```python
from build123d import *

# Parameters (mm, degrees)
SKETCH_1_W          = 65
SKETCH_1_H          = 70
EXTRUDE_1_DEPTH     = 4
SKETCH_2_R          = 2.1
SKETCH_2_R_2        = 1.575
SKETCH_2_R_3        = 14
CUT_EXTRUDE_1_DEPTH = 96.608577021
CUT_EXTRUDE_2_DEPTH = 96.608577021
FILLET_1_R          = 10


with BuildPart() as part:
    # 草图1 → 凸台-拉伸1 (new body)
    with BuildSketch(Plane.XY):
        with Locations((32.5, -35)):
            Rectangle(SKETCH_1_W, SKETCH_1_H)
    extrude(amount=EXTRUDE_1_DEPTH)

    # 草图2 → 切除-拉伸1 (cut, through all)
    with BuildSketch(Plane.XY.offset(4)):
        with Locations((25, -29.5)):
            Circle(SKETCH_2_R)
        with Locations((7.5, -47)):
            Circle(SKETCH_2_R)
        with Locations(Location((25, -64.5, 0), (0, 0, 180))):
            Circle(SKETCH_2_R)
        with Locations(Location((42.5, -47, 0), (0, 0, 180))):
            Circle(SKETCH_2_R)
        with Locations((40, -5)):
            Circle(SKETCH_2_R_2)
        with Locations(Location((50, -5, 0), (0, 0, 180))):
            Circle(SKETCH_2_R_2)
        with Locations((50, -15)):
            Circle(SKETCH_2_R_2)
        with Locations(Location((40, -15, 0), (0, 0, 180))):
            Circle(SKETCH_2_R_2)
        with Locations((25, -47)):
            Circle(SKETCH_2_R_3)
    extrude(amount=-CUT_EXTRUDE_1_DEPTH, mode=Mode.SUBTRACT)

    # 草图3 → 切除-拉伸2 (cut, through all)
    with BuildSketch(Plane(origin=(0, 0, 0), x_dir=(-1, 0, 0), z_dir=(0, 0, -1))):
        Polygon((-15, 0), (0, 0), (0, -35), align=None)
        Polygon((-65, 0), (-58, 0), (-65, -40), align=None)
    extrude(amount=-CUT_EXTRUDE_2_DEPTH, mode=Mode.SUBTRACT)

    # 圆角1
    fillet_1_edges = [part.edges().sort_by_distance(p)[0] for p in [
        (0, -35, 2),
        (15, 0, 2),
        (65, -40, 2),
        (58, 0, 2),
    ]]
    fillet(fillet_1_edges, radius=FILLET_1_R)


solid = part.part
```
The model under review builds one solid part; all positions refer to its coordinate system, in mm. Round coordinates to 2 decimals unless told otherwise and drop trailing zeros. Order: outer loops, then holes, each group sorted by start corner. A loop starts at its lowest first (then second) coordinate and runs counter-clockwise, first axis right, second up.
Item 1: Add section D-D, the plane y = -64.5. State the section outline as (x, z) points, and give its area (3 significant figures).
Working result:
outline: (0, 0) - (22.9, 0) - (22.9, 4) - (0, 4) - close; (27.1, 0) - (65, 0) - (65, 4) - (27.1, 4) - close
area: 243 mm2
Item 2: Add section A-A, the plane x = 7.5. State the section outline as (y, z) points.
Working result:
outline: (-70, 0) - (-49.1, 0) - (-49.1, 4) - (-70, 4) - close; (-44.9, 0) - (-17.5, 0) - (-17.5, 4) - (-44.9, 4) - close
Item 3: To check wall thickness, follow probe 1 along Y at (x, z) = (40, 0.25) (3 decimals); probe 2 along X at (y, z) = (-48, 3.1); probe 3 along Y at (x, z) = (25, 3). State the ranges of each line that lie inside material, in increasing order.
Working result:
probe 1: y = -70 to -16.575, -13.425 to -6.575, -3.425 to 0
probe 2: x = 0 to 5.65, 9.35 to 11.04, 38.96 to 40.65, 44.35 to 65
probe 3: y = -70 to -66.6, -62.4 to -61, -33 to -31.6, -27.4 to 0
Item 4: Add section C-C, the plane x = 25. State the section outline as (y, z) points, and give its area (3 significant figures).
Working result:
outline: (-70, 0) - (-66.6, 0) - (-66.6, 4) - (-70, 4) - close; (-62.4, 0) - (-61, 0) - (-61, 4) - (-62.4, 4) - close; (-33, 0) - (-31.6, 0) - (-31.6, 4) - (-33, 4) - close; (-27.4, 0) - (0, 0) - (0, 4) - (-27.4, 4) - close
area: 134 mm2
Item 5: Draft analysis for pull direction X (two halves, no side actions). For faces 1 (the flat face through (32, -34.5, 0)), 2 (the cylindrical face through (21.97, -60.67, 2.03)), 3 (the flat face through (6.524, -19.776, 1.972)), state which applies: released by +X, released by -X, zero draft, split by the parting line, or undercut.
Working result:
face 1: zero draft
face 2: undercut
face 3: released by -X
Item 6: For pin 1 (5.5 mm diameter, centred on x = 25, y = -29.5, fed in from -Z); pin 2 (3 mm diameter, centred on x = 50, y = -5, fed in from +Z); pin 3 (1 mm diameter, centred on y = -15, z = 2, fed in from -X), all flat-tipped, find the tip position at first contact; note any pin that passes through.
Working result:
pin 1: stops at z = 0
pin 2: passes through
pin 3: stops at x = 8.36
Item 7: Add section B-B, the plane y = -47. State the section outline as (x, z) points.
Working result:
outline: (0, 0) - (5.4, 0) - (5.4, 4) - (0, 4) - close; (9.6, 0) - (11, 0) - (11, 4) - (9.6, 4) - close; (39, 0) - (40.4, 0) - (40.4, 4) - (39, 4) - close; (44.6, 0) - (65, 0) - (65, 4) - (44.6, 4) - close
